Check sheet for the modelled part. Datum: model origin and axes. Units: mm. A direction names the side the tool comes from. Round coordinates to 2 decimals unless told otherwise and drop trailing zeros. Loops run counter-clockwise (first coordinate to the right, second up) from the corner with the lowest first, then second, coordinate; pieces in that order, holes last. Notation, with made-up numbers: (5, 52.25) - (17, 52.25) arc R17 ccw to (17, 73.25) - close; hole circle Ø5 at (17, 52). An arc over 180 degrees is marked (long way). Put each result on its own line as item: value. Start each with the question number.
Item 1: Section check D-D, the plane y = 12.75. Record the cut outline in (x, z).
Item 2: Draft check along Y on faces 1 (the flat face through (-3, 7, -6)), 2 (the cylindrical face through (-1.056, 9.524, 1.29)), 3 (the flat face through (-1, 0, 0)). Enter one of: pulls with the +Y half, pulls with the -Y half, needs draft (parallel to the pull), parting line crosses it, or undercut.
Item 3: Section check B-B, the plane z = -1. Record the cut outline in (x, y), and give its area (3 significant figures).
Item 4: Section check A-A, the plane y = 7.5. Record the cut outline in (x, z).
Item 5: Section check C-C, the plane x = 1.75. Record the cut outline in (y, z).
Item 6: Gauge pin test, flat ends, axial feed: pin 1 Ø5 at (y, z) = (8, 6) entering from +X; pin 2 Ø2 at (y, z) = (10, 6) entering from -X; pin 3 Ø0.6 at (x, y) = (-3.5, 10) entering from -Z; pin 4 Ø0.6 at (x, y) = (-4.5, 6) entering from +Z. Record the tip position at first contact, or that the pin passes through.
Item 7: Material ranges on line 1 along Y through (x, z) = (-3.5, 0); line 2 along Y through (x, z) = (-2.25, -1.5); line 3 along Z through (x, y) = (-0.75, 9), recorded low to high.
Item 8: Tool access check on faces 4 (the flat face through (-4, 7, -4)), 5 (the flat face through (-2, 7, 8)), 6 (the flat face through (-3, 7, 6)). Record the directions out of +Z, -Z, +X, -X, +Y, -Y that give a thin tool (end or side, any length) a straight path to the whole face; none if there is none.
Autodesk Inventor part; units mm, degrees
ref_plane "YZ Plane" through (0, 0, 0) normal (1, 0, 0) x (0, 1, 0)
ref_plane "XZ Plane" through (0, 0, 0) normal (0, 1, 0) x (-1, 0, 0)
ref_plane "XY Plane" through (0, 0, 0) normal (0, 0, 1) x (1, 0, 0)
sketch "Sketch1" plane through (0, 0, 0) normal (0, 1, 0) x (-1, 0, 0)
  line L0 (3, 8) -> (-3, 8)
  line L1 (-3, 8) -> (-3, -8)
  line L2 (-3, -8) -> (3, -8)
  line L3 (3, -8) -> (3, 8)
  line L4 (3, 8) -> (-3, -8) construction
  line L5 (-3, 8) -> (3, -8) construction
  line L6 (5, 4) -> (1, 4)
  line L7 (1, 4) -> (1, -4)
  line L8 (1, -4) -> (5, -4)
  line L9 (5, -4) -> (5, 4)
  line L10 (5, 4) -> (1, -4) construction
  line L11 (1, 4) -> (5, -4) construction
  line L12 (0, 8) -> (-3, 4.5)
  line L13 (-3, -4.5) -> (0, -8)
  point P0 (0, 0)
  point P1 (3, 0)
  point P2 (-3, 0)
  point P3 (3, 4)
  point P4 (3, -4)
  dimension "d0" = 6
  dimension "d1" = 16
  dimension "d2" = 4
  dimension "d3" = 8
  dimension "d4" = 3
  dimension "d5" = 3
  dimension "d6" = 9
  dimension "d7" = 4.5
extrude "Extrusion1" add sketch "Sketch1" along normal blind 15 contours L3 L6 L7 L8 L2 L13 L1 L12 L0 | L6 L9 L8 L3 | L3 L8 L7 L6
sketch "Sketch2" plane through (-5, 0, -4) normal (-1, 0, 0) x (0, 0, 1)
  circle A0 centre (4, 7.5) radius 2.4
  line L0 (0, 0) -> (8, 0)
  line L1 (8, 0) -> (8, 15)
  point P0 (4, 0)
  dimension "d10" = 4.8
  dimension "d11" = 7.5
  dimension "d12" = 4
extrude "Extrusion2" cut sketch "Sketch2" against normal through all
properties part number "drazkaVel"
Check result:
1. outline: (-5, -4) - (-3, -4) - (-3, -8) - (0, -8) - (3, -4.5) - (3, 4.5) - (0, 8) - (-3, 8) - (-3, 4) - (-5, 4) - close
2. face 1: needs draft
2. face 2: undercut
2. face 3: pulls with the -Y half
3. outline: (-5, 0) - (3, 0) - (3, 5.32) - (-5, 5.32) - close; (-5, 9.68) - (3, 9.68) - (3, 15) - (-5, 15) - close
3. area: 85.1 mm²
4. outline: (-5, -4) - (-3, -4) - (-3, -8) - (0, -8) - (3, -4.5) - (3, -2.4) - (-5, -2.4) - close; (-5, 2.4) - (3, 2.4) - (3, 4.5) - (0, 8) - (-3, 8) - (-3, 4) - (-5, 4) - close
5. outline: (0, -5.96) - (15, -5.96) - (15, 5.96) - (0, 5.96) - close; hole circle Ø4.8 at (7.5, 0)
6. pin 1: x = 3
6. pin 2: x = -3
6. pin 3: z = -4
6. pin 4: z = 4
7. line 1: 0 to 5.1, 9.9 to 15
7. line 2: 0 to 5.63, 9.37 to 15
7. line 3: -8 to -1.87, 1.87 to 8
8. face 4: -Z, -X, +Y, -Y
8. face 5: +Z, +X, -X, +Y, -Y
8. face 6: +Z, -X, +Y, -Y
